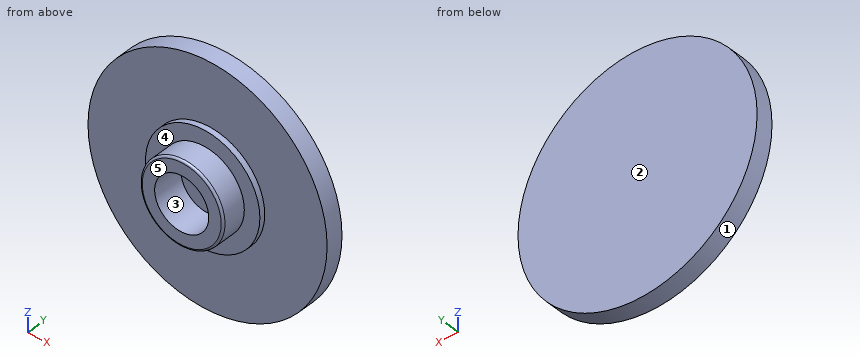
```python
from build123d import *

# Parameters (mm, degrees)
F0_R     = 11.5
F1_DEPTH = 1.7
F2_R     = 5.5
F3_DEPTH = 2.25
F4_R     = 4
F5_DEPTH = 4.65
F6_R     = 0.2
F7_R     = 2.6
F8_DEPTH = 3


with BuildPart() as f1:
    # F0 (on Front) → F1 (new body)
    with BuildSketch(Plane.XZ):
        Circle(F0_R)
    extrude(amount=F1_DEPTH)

    # F2 (on Front) → F3 (join)
    with BuildSketch(Plane.XZ):
        Circle(F2_R)
    extrude(amount=F3_DEPTH)

    # F4 (on Front) → F5 (join)
    with BuildSketch(Plane.XZ):
        Circle(F4_R)
    extrude(amount=F5_DEPTH)

    # F6
    f6_edges = [f1.edges().sort_by_distance(p)[0] for p in [
        (-4, -4.65, 0),
    ]]
    fillet(f6_edges, radius=F6_R)

    # F7 (on face) → F8 (cut)
    with BuildSketch(Plane.XZ.offset(4.65)):
        Circle(F7_R)
    extrude(amount=-F8_DEPTH, mode=Mode.SUBTRACT)


solid = f1.part
```
Design review of the part built by this model. Coordinates are the model's own, in mm. Face numbers are marked on the shaded views. A direction names the side the tool comes from. Give positions to 0.01 mm unless a question says otherwise; leave off trailing zeros. Write each loop counter-clockwise with the first axis right and the second up, starting at its lowest first coordinate (ties: lowest second). Pieces come first, ordered by that corner, then holes. Notation, with made-up numbers: (-14, 87) - (15, 87) arc R14 ccw to (15, 97) - close; hole circle Ø7 at (53.5, 51). An arc over 180 degrees is marked (long way). Return JSON: item names as keys, results as strings. Group by question number.
(1) We need section D-D, the plane y = -0.6. Give the boundary of the cut face in (x, z), then the cut area to 3 significant figures.
(2) Insertion check: pin 1 (2 mm diameter, centred on y = -0.5, z = -6.5, fed in from +X); pin 2 (2 mm diameter, centred on y = -0.5, z = -4.5, fed in from -X); pin 3 (1.5 mm diameter, centred on x = 1, y = -2, fed in from +Z). Each pin has a flat end and moves straight along its axis. Give the tip position at first contact, or say it passes through.
(3) We need section A-A, the plane z = 0. Give the boundary of the cut face in (x, y).
(4) To check wall thickness, follow probe 1 along Z at (x, y) = (0, -3.3); probe 2 along Y at (x, z) = (2, 4.5); probe 3 along Y at (x, z) = (-6.5, 4.25). State the ranges of each line that lie inside material, in increasing order.
(5) Machinability: for the marked faces 4 and 5, which of the approach directions +Z, -Z, +X, -X, +Y, -Y give a long, thin tool a straight path to every point of the face, cutting with its end or side? Answer none if there is none.
(6) We need section C-C, the plane x = 0. Give the boundary of the cut face in (y, z).
(7) Mouldability with a two-part tool opening along X and no side actions: class the marked faces 1, 2 and 3 as +X half, -X half, draft (parallel to the pull), parting line (faces both ways), or undercut.
(8) We need section B-B, the plane y = -3.25. Give the boundary of the cut face in (x, z).
Reported:
{
 "1": {"outline": "circle Ø23 at (0, 0)", "area": "415 mm2"},
 "2": {"pin 1": "stops at x = 10.1", "pin 2": "stops at x = -10.95", "pin 3": "stops at z = 11.5"},
 "3": {"outline": "(-11.5, -1.7) - (-5.5, -1.7) - (-5.5, -2.25) - (-4, -2.25) - (-4, -4.45) arc R0.2 ccw to (-3.8, -4.65) - (-2.6, -4.65) - (-2.6, -1.65) - (2.6, -1.65) - (2.6, -4.65) - (3.8, -4.65) arc R0.2 ccw to (4, -4.45) - (4, -2.25) - (5.5, -2.25) - (5.5, -1.7) - (11.5, -1.7) - (11.5, 0) - (-11.5, 0) - close"},
 "4": {"probe 1": "z = -4 to -2.6, 2.6 to 4", "probe 2": "y = -2.25 to 0", "probe 3": "y = -1.7 to 0"},
 "5": {"face 4": "-Y", "face 5": "+Z, -Z, +X, -X, -Y"},
 "6": {"outline": "(-4.65, -3.8) arc R0.2 ccw to (-4.45, -4) - (-2.25, -4) - (-2.25, -5.5) - (-1.7, -5.5) - (-1.7, -11.5) - (0, -11.5) - (0, 11.5) - (-1.7, 11.5) - (-1.7, 5.5) - (-2.25, 5.5) - (-2.25, 4) - (-4.45, 4) arc R0.2 ccw to (-4.65, 3.8) - (-4.65, 2.6) - (-1.65, 2.6) - (-1.65, -2.6) - (-4.65, -2.6) - close"},
 "7": {"face 1": "parting line", "face 2": "draft", "face 3": "undercut"},
 "8": {"outline": "circle Ø8 at (0, 0); hole circle Ø5.2 at (0, 0)"}
}
